```python
from build123d import *

# Parameters (mm, degrees)
F1_DEPTH  = 67.5
F3_W      = 49.2
F3_H      = 49.2
F4_DEPTH  = 28
F6_W      = 57.5
F6_H      = 48
F7_DEPTH  = 40
F9_DEPTH  = 5
F10_R     = 12.5
F11_DEPTH = 20
F13_R     = 34.5
F14_DEPTH = 37.5
F16_W     = 52.5
F16_H     = 48
F17_DEPTH = 25
F18_R     = 24.6
F19_DEPTH = 20


with BuildPart() as f1:
    # F0 (on Front) → F1 (new body)
    with BuildSketch(Plane.XZ):
        with BuildLine():
            ThreePointArc((-35.5098846553, 0.5000012368), (-7.5727771152, 12.0657876083), (4, 40))
            ThreePointArc((4, 40), (2.8997637092, 49.2578694674), (-0.3396530165, 58))
            ThreePointArc((-0.3396530165, 58), (-69.1964570083, 60.6106473718), (-35.5098846553, 0.5000012368))
        make_face()
        with BuildLine():
            ThreePointArc((-0.3396530165, 58), (2.8997637092, 49.2578694674), (4, 40))
            ThreePointArc((4, 40), (-7.5727771152, 12.0657876083), (-35.5098846553, 0.5000012368))
            Line((-35.5098846553, 0.5000012368), (0, 0))
            Line((0, 0), (75, 0))
            Line((75, 0), (75, 80))
            Line((75, 80), (41, 80))
            Line((41, 80), (41, 58))
            Line((41, 58), (-0.3396530165, 58))
        make_face()
    extrude(amount=-F1_DEPTH)

    # F3 (on offset) → F4 (cut)
    with BuildSketch(Plane.YZ.offset(75)):
        with Locations((32.5, 40)):
            Rectangle(F3_W, F3_H)
    extrude(amount=-F4_DEPTH, mode=Mode.SUBTRACT)

    # F6 (on offset) → F7 (cut)
    with BuildSketch(Plane.YZ.offset(47)):
        with Locations((33.75, 29)):
            Rectangle(F6_W, F6_H)
    extrude(amount=-F7_DEPTH, mode=Mode.SUBTRACT)

    # F8 (on face) → F9 (cut)
    with BuildSketch(Plane.XZ):
        with BuildLine():
            ThreePointArc((-27.0960278356, 0.3815289056), (-4.0308812273, 14.5059896511), (5, 40))
            ThreePointArc((5, 40), (3.9309299575, 49.2440122613), (0.7801598673, 58))
            Line((0.7801598673, 58), (-0.3396530165, 58))
            ThreePointArc((-0.3396530165, 58), (-69.1964570083, 60.6106473718), (-35.5098846553, 0.5000012368))
            Line((-35.5098846553, 0.5000012368), (-27.0960278356, 0.3815289056))
        make_face()
    extrude(amount=-F9_DEPTH, mode=Mode.SUBTRACT)

    # F10 (on face) → F11 (cut)
    with BuildSketch(Plane.XZ.offset(-5)):
        with Locations((-35.5, 40)):
            Circle(F10_R)
    extrude(amount=-F11_DEPTH, mode=Mode.SUBTRACT)

    # F13 (on offset) → F14 (cut)
    with BuildSketch(Plane.XZ.offset(-25)):
        with Locations((-35.5, 40)):
            Circle(F13_R)
    extrude(amount=-F14_DEPTH, mode=Mode.SUBTRACT)

    # F16 (on offset) → F17 (cut)
    with BuildSketch(Plane.YZ.offset(7)):
        with Locations((36.25, 29)):
            Rectangle(F16_W, F16_H)
    extrude(amount=-F17_DEPTH, mode=Mode.SUBTRACT)

    # F18 (on Top) → F19 (cut)
    with BuildSketch(Plane.XY):
        with Locations((-45, 32.5)):
            Circle(F18_R)
        with Locations((35, 32.5)):
            Circle(F18_R)
    extrude(amount=F19_DEPTH, mode=Mode.SUBTRACT)


solid = f1.part
```
For this review, take the finished solid that the model builds, in its own axes (mm). A direction names the side the tool comes from. Give positions to 0.01 mm unless a question says otherwise; leave off trailing zeros. Write each loop counter-clockwise with the first axis right and the second up, starting at its lowest first coordinate (ties: lowest second). Pieces come first, ordered by that corner, then holes.
Item 1: Take a section at D-D (x = -16). Give the boundary of the cut face in (y, z), and give its area (3 significant figures).
Item 2: Take a section at B-B (z = 72). Give the boundary of the cut face in (x, y), and give its area (3 significant figures).
Item 3: Take a section at C-C (y = 39.5). Give the boundary of the cut face in (x, z).
Item 4: The part is to be moulded in two halves that separate along Y. For faces 5 (the face through (-26.653, 16.112, 10.006)), 6 (the face through (-1, 67.5, 41)), 7 (the face through (21, 33, 58)), say which applies: +Y half, -Y half, draft (parallel to the pull), parting line (faces both ways), or undercut.
Item 5: Insertion check: P1, Ø11, axis at y = 25.5, z = 73.5, coming from the -X side; P2, Ø9.5, axis at y = 58, z = 27, coming from the -X side; P3, Ø8, axis at y = 53.5, z = 64, coming from the -X side. Each pin has a flat end and moves straight along its axis. Give the tip position at first contact, or say it passes through.
Item 6: Machinability: for faces 1 (the face through (45, 56, 0)), 2 (the face through (-45.42, 14.86, 32.394)), 3 (the face through (47, 7, 24)), 4 (the face through (64, 32, 15.4)), which of the approach directions +Z, -Z, +X, -X, +Y, -Y give a long, thin tool a straight path to every point of the face, cutting with its end or side? Answer none if there is none.
Item 7: Wall thickness on probe 1 along Y at (x, z) = (-45, 12.75); probe 2 along Z at (x, y) = (67, 49); probe 3 along Y at (x, z) = (-49, 55): over which ranges is each line inside the solid? List them lowest first.
Item 8: Take a section at A-A (y = 19). Give the boundary of the cut face in (x, z), and give its area (3 significant figures).
Established:
1. outline: (0, 0.23) - (67.5, 0.23) - (67.5, 74.35) - (5, 74.35) - (5, 4.5) - (0, 4.5) - close; hole (10, 5) - (62.5, 5) - (62.5, 68.46) - (25, 68.46) - (25, 53) - (10, 53) - close
1. area: 1,550 mm2
2. outline: (-58.66, 5) - (-12.34, 5) - (-12.34, 67.5) - (-58.66, 67.5) - close; (41, 0) - (75, 0) - (75, 67.5) - (41, 67.5) - close; hole (-48.39, 25) - (-22.61, 25) - (-22.61, 62.5) - (-48.39, 62.5) - close
2. area: 4,220 mm2
3. outline: (-68.58, 18.42) - (-68.58, 20) - (-63.61, 20) arc R34.5 cw (long way) to (-3.54, 53) - (47, 53) - (47, 64.6) - (75, 64.6) - (75, 80) - (41, 80) - (41, 58) - (-0.34, 58) arc R39.5 ccw (long way) to start; (-21.42, 0.3) - (0, 0) - (11.42, 0) - (11.42, 5) - (-18, 5) - (-18, 10.27) arc R34.5 cw to (-21.42, 8.51) - close; (58.58, 0) - (75, 0) - (75, 15.4) - (58.58, 15.4) - close
4. face 5: undercut
4. face 6: +Y half
4. face 7: draft
5. P1: stops at x = -63.36
5. P2: stops at x = -74.13
5. P3: stops at x = -69.56
6. face 1: -Z, +X, -X, +Y, -Y
6. face 2: -Y
6. face 3: none
6. face 4: +X
7. probe 1: y = 5 to 7.9, 62.5 to 67.5
7. probe 2: z = 0 to 15.4, 64.6 to 80
7. probe 3: y = 5 to 25, 62.5 to 67.5
8. outline: (-65.56, 14.38) - (-65.56, 20) - (-24.44, 20) - (-24.44, 0.34) - (0, 0) - (14.44, 0) - (14.44, 5) - (-18, 5) - (-18, 53) - (47, 53) - (47, 64.6) - (75, 64.6) - (75, 80) - (41, 80) - (41, 58) - (-0.34, 58) arc R39.5 ccw (long way) to start; (55.56, 0) - (75, 0) - (75, 15.4) - (55.56, 15.4) - close; hole circle Ø25 at (-35.5, 40)
8. area: 4,180 mm2
